Read the model definition and answer for the solid it produces. Units are mm, in the model's axes. Face numbers are marked on the shaded views. A direction names the side the tool comes from. Coordinates: 2 decimals unless noted, no trailing zeros. Write each loop counter-clockwise with the first axis right and the second up, starting at its lowest first coordinate (ties: lowest second). Pieces come first, ordered by that corner, then holes.
1) The part is cut by section C-C (y = -11.25). Determine the outline of the cut face in (x, z), then the cut area to 3 significant figures.
2) The part is cut by section D-D (z = -4.5). Determine the outline of the cut face in (x, y), then the cut area to 3 significant figures.
3) The part is cut by section A-A (z = 1.25). Determine the outline of the cut face in (x, y).
4) The part is cut by section B-B (x = 0.5). Determine the outline of the cut face in (y, z), then the cut area to 3 significant figures.
5) Which of the six approach directions +Z, -Z, +X, -X, +Y, -Y give full straight-line access (tool end or side, diameter ignored) to the marked faces 1, 2 and 3?
6) Determine the mould class of the marked faces 4, 5 and 6 for opening direction X: +X half, -X half, draft (parallel to the pull), parting line (faces both ways), or undercut.
7) Each of these flat-tipped pins is pushed along its axis until it touches: pin 1 Ø3.5 at (x, y) = (0, 0) entering from -Z; pin 2 Ø3 at (x, y) = (2, -11) entering from +Z; pin 3 Ø1 at (y, z) = (-11.5, -2.5) entering from -X. Where does it stop, or does it pass through?
8) Find the intervals of material crossed by line 1 (Y direction, x = 0, z = -1.1); line 2 (Y direction, x = 0, z = -2.15); line 3 (Z direction, x = -3.5, y = -10.25), in increasing order.
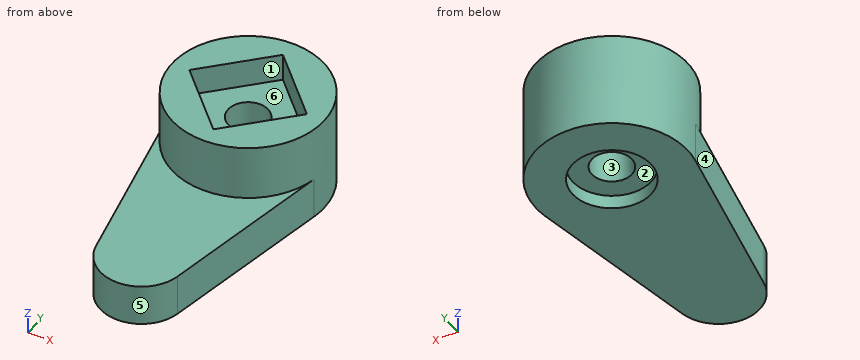
from build123d import *

# Parameters (mm, degrees)
F0_R          = 5.5
F1_DEPTH      = 5
F1_DEPTH_BACK = 2
F3_DEPTH      = 2
F5_START      = -2
F5_DEPTH      = 3
F7_START      = -4
F6_R          = 2.85
F7_DEPTH      = 21
F8_R          = 1.45
F9_DEPTH      = 25
F9_DEPTH_BACK = 25


with BuildPart() as f1:
    # F0 (on Top) → F1 (new body, two sides)
    with BuildSketch(Plane.XY) as f1_sk:
        Circle(F0_R)
    extrude(amount=-F1_DEPTH)
    extrude(f1_sk.sketch, amount=F1_DEPTH_BACK)

    # F2 (on Top) → F3 (cut)
    with BuildSketch(Plane.XY):
        Polygon((4.2426406871, 0), (0, 4.2426406871), (-4.2426406871, 0), (0, -4.2426406871), align=None)
    extrude(amount=F3_DEPTH, mode=Mode.SUBTRACT)

    # F4 (on Top) → F5 (join)
    with BuildSketch(Plane.XY.offset(F5_START)):
        with BuildLine():
            Line((-5.3973407325, -1.0576923077), (-2.9440040359, -13.5769230769))
            ThreePointArc((-2.9440040359, -13.5769230769), (0, -16), (2.9440040359, -13.5769230769))
            Line((2.9440040359, -13.5769230769), (5.3973407325, -1.0576923077))
            ThreePointArc((5.3973407325, -1.0576923077), (0, 5.5), (-5.3973407325, -1.0576923077))
        make_face()
    extrude(amount=-F5_DEPTH)

    # F6 (on Top) → F7 (cut)
    with BuildSketch(Plane.XY.offset(F7_START)):
        Circle(F6_R)
    extrude(amount=-F7_DEPTH, mode=Mode.SUBTRACT)

    # F8 (on Top) → F9 (cut, two sides)
    with BuildSketch(Plane.XY) as f9_sk:
        Circle(F8_R)
    extrude(amount=-F9_DEPTH, mode=Mode.SUBTRACT)
    extrude(f9_sk.sketch, amount=F9_DEPTH_BACK, mode=Mode.SUBTRACT)


solid = f1.part
Reported:
1. outline: (-3.4, -5) - (3.4, -5) - (3.4, -2) - (-3.4, -2) - close
1. area: 20.4 mm2
2. outline: (-5.4, -1.06) - (-2.94, -13.58) arc R3 ccw to (2.94, -13.58) - (5.4, -1.06) arc R5.5 ccw (long way) to start; hole circle Ø5.7 at (0, 0)
2. area: 149 mm2
3. outline: circle Ø11 at (0, 0); hole (-4.24, 0) - (0, -4.24) - (4.24, 0) - (0, 4.24) - close
4. outline: (-15.96, -5) - (-2.81, -5) - (-2.81, -4) - (-1.36, -4) - (-1.36, 0) - (-3.74, 0) - (-3.74, 2) - (-5.48, 2) - (-5.48, -2) - (-15.96, -2) - close; (1.36, -4) - (2.81, -4) - (2.81, -5) - (5.48, -5) - (5.48, 2) - (3.74, 2) - (3.74, 0) - (1.36, 0) - close
4. area: 76.7 mm2
5. face 1: +Z
5. face 2: -Z
5. face 3: +Z, -Z
6. face 4: -X half
6. face 5: parting line
6. face 6: undercut
7. pin 1: stops at z = -4
7. pin 2: stops at z = -2
7. pin 3: stops at x = -3.45
8. line 1: y = -5.5 to -1.45, 1.45 to 5.5
8. line 2: y = -16 to -1.45, 1.45 to 5.5
8. line 3: z = -5 to -2
